Here's how the part is built. I have some questions about the finished solid (model axes, mm). A direction names the side the tool comes from. Give positions to 0.01 mm unless a question says otherwise; leave off trailing zeros. Loops run counter-clockwise (first coordinate to the right, second up) from the corner with the lowest first, then second, coordinate; pieces in that order, holes last.
Q1. If we section it at A-A (y = 2): Please give me the cut outline in (x, z), plus the area to 3 significant figures.
Q2. I need wall thicknesses on line 1 (Z direction, x = -0.5, y = -1.75); line 2 (X direction, y = -3, z = -23); line 3 (X direction, y = -1.25, z = -29). Which ranges of each line are inside material? Lowest first, please.
Q3. If we section it at B-B (x = -1): Please give me the cut outline in (y, z) (3 decimals).
Q4. For faces 1 (the face through (1.967, 0, -26)), 2 (the face through (0, 0, -35.776)), which set-ups out of +Z, -Z, +X, -X, +Y, -Y let a thin tool reach every point of the face, with its end or its side?
Q5. We'd pull the mould along X, two halves only. Please class faces 3 (the face through (-0.11, -0.04, -30.97)), 4 (the face through (0, 3.175, 1)), 5 (the face through (-2.489, 0, -27)), 6 (the face through (5.08, 0, -1)): +X half, -X half, draft (parallel to the pull), parting line (faces both ways), or undercut.
from build123d import *

# Parameters (mm, degrees)
F0_W     = 10.16
F0_H     = 71.552346
F1_DEPTH = 3.175


with BuildPart() as f1:
    # F0 (on Front) → F1 (new body, symmetric)
    with BuildSketch(Plane.XZ):
        Rectangle(F0_W, F0_H)
        with BuildLine():
            ThreePointArc((-2.489432, -24.29621), (-0.303735, -21.756134), (1.967174, -24.220324))
            Line((1.967174, -24.220324), (1.967174, -28.548131))
            ThreePointArc((1.967174, -28.548131), (-0.15872, -30.974596), (-2.489432, -28.744139))
            Line((-2.489432, -28.744139), (-2.489432, -24.29621))
        make_face(mode=Mode.SUBTRACT)
    extrude(amount=F1_DEPTH, both=True)


solid = f1.part
Check sheet entries:
1. outline: (-5.08, -35.78) - (5.08, -35.78) - (5.08, 35.78) - (-5.08, 35.78) - close; hole (-2.49, -28.74) arc R2.23 ccw (long way) to (1.97, -28.55) - (1.97, -24.22) arc R2.24 ccw (long way) to (-2.49, -24.3) - close
1. area: 690 mm2
2. line 1: z = -35.78 to -30.96, -21.77 to 35.78
2. line 2: x = -5.08 to -2.27, 1.74 to 5.08
2. line 3: x = -5.08 to -2.47, 1.96 to 5.08
3. outline: (-3.175, -35.776) - (3.175, -35.776) - (3.175, -30.849) - (-3.175, -30.849) - close; (-3.175, -21.879) - (3.175, -21.879) - (3.175, 35.776) - (-3.175, 35.776) - close
4. face 1: +Y, -Y
4. face 2: -Z, +X, -X, +Y, -Y
5. face 3: undercut
5. face 4: draft
5. face 5: undercut
5. face 6: +X half
